from build123d import *

# Parameters (mm, degrees)
SKETCH_1_W      = 74.6
SKETCH_1_H      = 42
EXTRUDE_1_DEPTH = 1
FILLET_1_R      = 2
SKETCH_2_W      = 84.6
SKETCH_2_H      = 47
EXTRUDE_2_DEPTH = 1
FILLET_2_R      = 1


with BuildPart() as part:
    # Эскиз1 → Бобышка-Вытянуть1 (new body)
    with BuildSketch(Plane(origin=(0, 0, 0), x_dir=(1, 0, 0), z_dir=(0, 1, 0))):
        Rectangle(SKETCH_1_W, SKETCH_1_H)
    extrude(amount=EXTRUDE_1_DEPTH)

    # Скругление1
    fillet_1_edges = [part.edges().sort_by_distance(p)[0] for p in [
        (-37.3, 0.5, -21),
        (37.3, 0.5, -21),
    ]]
    fillet(fillet_1_edges, radius=FILLET_1_R)

    # Эскиз2 → Бобышка-Вытянуть2 (add)
    with BuildSketch(Plane.XZ):
        with Locations((0, -2.5)):
            Rectangle(SKETCH_2_W, SKETCH_2_H)
    extrude(amount=EXTRUDE_2_DEPTH)

    # Скругление2
    fillet_2_edges = [part.edges().sort_by_distance(p)[0] for p in [
        (-42.3, -0.5, -26),
        (42.3, -0.5, -26),
    ]]
    fillet(fillet_2_edges, radius=FILLET_2_R)


solid = part.part
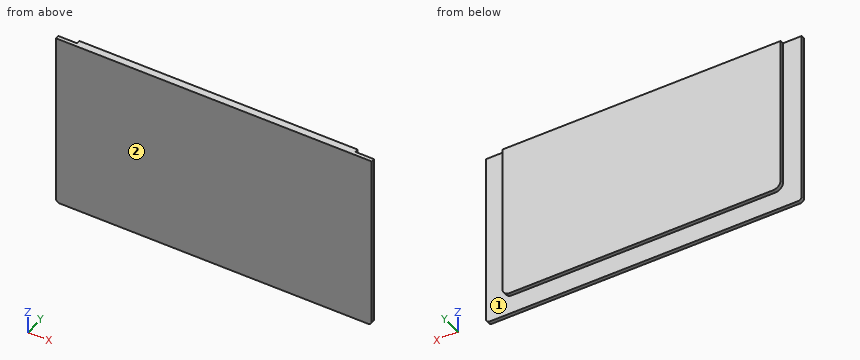
Design review of the part built by this model. Coordinates are the model's own, in mm. Face numbers are marked on the shaded views. A direction names the side the tool comes from. Round coordinates to 2 decimals unless told otherwise and drop trailing zeros. Loops run counter-clockwise (first coordinate to the right, second up) from the corner with the lowest first, then second, coordinate; pieces in that order, holes last. Notation, with made-up numbers: (51.5, 24.25) -> (75.5, 24.25) arc R24 ccw to (75.5, 54.25) -> close; hole circle Ø9 at (4, 43.5). An arc over 180 degrees is marked (long way). Use one line per item in the form item = value. Start each with the question number.
Q1. For pin 1 Ø0.5 at (x, y) = (5, 0.5) entering from -Z, flat-tipped, find the tip position at first contact; note if it passes through.
Q2. Machinability: for the marked faces 1 and 2, which of the approach directions +Z, -Z, +X, -X, +Y, -Y give a long, thin tool a straight path to every point of the face, cutting with its end or side? Answer none if there is none.
Q3. We need section C-C on x = 3. Give the boundary of the cut face in (y, z), then the cut area to 3 significant figures.
Q4. We need section A-A on z = -6. Give the boundary of the cut face in (x, y), then the cut area to 3 significant figures.
Q5. We need section B-B on y = 0.65. Give the boundary of the cut face in (x, z), then the cut area to 3 significant figures.
Q6. Wall thickness on line 1 along Z through (x, y) = (21.5, 0.9); line 2 along X through (y, z) = (0.2, 16); line 3 along Y through (x, z) = (-37, -22.5): over which ranges is each line inside the solid? List them lowest first. Write a range as [from, to].
Calculated:
q1.pin_1 = -21
q2.face_1 = -Z, +Y
q2.face_2 = +Z, -Z, +X, -X, -Y
q3.outline = (-1, -26) -> (0, -26) -> (0, -21) -> (1, -21) -> (1, 21) -> (-1, 21) -> close
q3.area = 89.0 mm²
q4.outline = (-42.3, -1) -> (42.3, -1) -> (42.3, 0) -> (37.3, 0) -> (37.3, 1) -> (-37.3, 1) -> (-37.3, 0) -> (-42.3, 0) -> close
q4.area = 159 mm²
q5.outline = (-37.3, -19) arc R2 ccw to (-35.3, -21) -> (35.3, -21) arc R2 ccw to (37.3, -19) -> (37.3, 21) -> (-37.3, 21) -> close
q5.area = 3,130 mm²
q6.line_1 = [-21, 21]
q6.line_2 = [-37.3, 37.3]
q6.line_3 = [-1, 0]
